Can you work these out from the model? Positions are in its coordinate system, mm. A direction names the side the tool comes from. Give positions to 0.01 mm unless a question says otherwise; leave off trailing zeros. Order: outer loops, then holes, each group sorted by start corner. A loop starts at its lowest first (then second) coordinate and runs counter-clockwise, first axis right, second up. Notation, with made-up numbers: (63.5, 84.5) - (116.5, 84.5) arc R20 ccw to (116.5, 99.5) - close; hole circle Ø1 at (65, -10). An arc over 180 degrees is marked (long way). Answer as CSV lines item,"result".
```python
from build123d import *

# Parameters (mm, degrees)
F0_W         = 35
F0_H         = 5
F1_DEPTH     = 1
F2_DEPTH     = 1.2
F3_W         = 5
F3_H         = 85
F4_DEPTH     = 2
F5_T4_DEPTH  = 99.1421356237
F5_T9_DEPTH  = 99.1421356237
F5_T14_DEPTH = 99.1421356237
F5_T19_DEPTH = 99.1421356237
F5_T24_DEPTH = 99.1421356237
F5_T29_DEPTH = 99.1421356237
F5_T34_DEPTH = 99.1421356237
F5_T39_DEPTH = 99.1421356237
F6_R         = 5


# Not quite as in the source:
# - a fillet or chamfer that OpenCascade refuses, or shapes differently, is made with other operations: its cross-section is extruded or revolved along the edge and cut away or added


with BuildPart() as f1:
    # F0 (on Top) → F1 (new body)
    with BuildSketch(Plane.XY):
        Polygon((-19.95, -49.95), (19.95, -49.95), (19.95, 49.95), (17.5, 49.95), (17.5, 44.95), (-17.5, 44.95), (-17.5, 49.95), (-19.95, 49.95), align=None)
        with Locations((0, 47.45)):
            Rectangle(F0_W, F0_H)
    extrude(amount=F1_DEPTH)

    # F0 (on Top) → F2 (join)
    with BuildSketch(Plane.XY):
        with Locations((0, 52.45)):
            Rectangle(F0_W, F0_H)
        with Locations((0, 47.45)):
            Rectangle(F0_W, F0_H)
    extrude(amount=-F2_DEPTH)

    # F3 (on face) → F4 (join)
    with BuildSketch(Plane.XY):
        with Locations((-12.45, 2.55)):
            Rectangle(F3_W, F3_H)
        with Locations((12.45, 2.55)):
            Rectangle(F3_W, F3_H)
    extrude(amount=-F4_DEPTH)

    # F5: fillet of radius 3 on 4 edges, made by hand


with BuildPart() as f5_tool2:
    # F5_s3 → F5_t4 (new body)
    with BuildSketch(Plane.XZ.offset(-52.1210678119)):
        with BuildLine():
            ThreePointArc((-14.95, 0), (-13.8536236828, -1.4494897428), (-12.1215728753, -2))
            Line((-12.1215728753, -2), (-14.95, -2))
            Line((-14.95, -2), (-14.95, 0))
        make_face()
    extrude(amount=F5_T4_DEPTH)

    split(bisect_by=Plane.XY.offset(-1.2), keep=Keep.BOTTOM)


with BuildPart() as f1_1:
    add(f1.part)

    # F5_t1: cut F5_tool2
    add(f5_tool2.part, mode=Mode.SUBTRACT)


with BuildPart() as f5_tool7:
    # F5_s8 → F5_t9 (new body)
    with BuildSketch(Plane.XZ.offset(-52.1210678119)):
        with BuildLine():
            ThreePointArc((-14.95, 0), (-13.8536236828, -1.4494897428), (-12.1215728753, -2))
            Line((-12.1215728753, -2), (-14.95, -2))
            Line((-14.95, -2), (-14.95, 0))
        make_face()
    extrude(amount=F5_T9_DEPTH)

    split(bisect_by=Plane.XZ.offset(-44.95), keep=Keep.TOP)


with BuildPart() as f1_2:
    add(f1_1.part)

    # F5_t6: cut F5_tool7
    add(f5_tool7.part, mode=Mode.SUBTRACT)


with BuildPart() as f5_tool12:
    # F5_s13 → F5_t14 (new body)
    with BuildSketch(Plane.XZ.offset(47.0210678119)):
        with BuildLine():
            ThreePointArc((-9.95, 0), (-11.0463763172, -1.4494897428), (-12.7784271247, -2))
            Line((-12.7784271247, -2), (-9.95, -2))
            Line((-9.95, -2), (-9.95, 0))
        make_face()
    extrude(amount=-F5_T14_DEPTH)

    split(bisect_by=Plane.XZ.offset(-44.95), keep=Keep.TOP)


with BuildPart() as f1_3:
    add(f1_2.part)

    # F5_t11: cut F5_tool12
    add(f5_tool12.part, mode=Mode.SUBTRACT)


with BuildPart() as f5_tool17:
    # F5_s18 → F5_t19 (new body)
    with BuildSketch(Plane.XZ.offset(47.0210678119)):
        with BuildLine():
            ThreePointArc((-9.95, 0), (-11.0463763172, -1.4494897428), (-12.7784271247, -2))
            Line((-12.7784271247, -2), (-9.95, -2))
            Line((-9.95, -2), (-9.95, 0))
        make_face()
    extrude(amount=-F5_T19_DEPTH)

    split(bisect_by=Plane.XY.offset(-1.2), keep=Keep.BOTTOM)


with BuildPart() as f1_4:
    add(f1_3.part)

    # F5_t16: cut F5_tool17
    add(f5_tool17.part, mode=Mode.SUBTRACT)


with BuildPart() as f5_tool22:
    # F5_s23 → F5_t24 (new body)
    with BuildSketch(Plane.XZ.offset(47.0210678119)):
        with BuildLine():
            ThreePointArc((14.95, 0), (13.8536236828, -1.4494897428), (12.1215728753, -2))
            Line((12.1215728753, -2), (14.95, -2))
            Line((14.95, -2), (14.95, 0))
        make_face()
    extrude(amount=-F5_T24_DEPTH)

    split(bisect_by=Plane.XZ.offset(-44.95), keep=Keep.TOP)


with BuildPart() as f1_5:
    add(f1_4.part)

    # F5_t21: cut F5_tool22
    add(f5_tool22.part, mode=Mode.SUBTRACT)


with BuildPart() as f5_tool27:
    # F5_s28 → F5_t29 (new body)
    with BuildSketch(Plane.XZ.offset(47.0210678119)):
        with BuildLine():
            ThreePointArc((14.95, 0), (13.8536236828, -1.4494897428), (12.1215728753, -2))
            Line((12.1215728753, -2), (14.95, -2))
            Line((14.95, -2), (14.95, 0))
        make_face()
    extrude(amount=-F5_T29_DEPTH)

    split(bisect_by=Plane.XY.offset(-1.2), keep=Keep.BOTTOM)


with BuildPart() as f1_6:
    add(f1_5.part)

    # F5_t26: cut F5_tool27
    add(f5_tool27.part, mode=Mode.SUBTRACT)


with BuildPart() as f5_tool32:
    # F5_s33 → F5_t34 (new body)
    with BuildSketch(Plane.XZ.offset(-52.1210678119)):
        with BuildLine():
            ThreePointArc((9.95, 0), (11.0463763172, -1.4494897428), (12.7784271247, -2))
            Line((12.7784271247, -2), (9.95, -2))
            Line((9.95, -2), (9.95, 0))
        make_face()
    extrude(amount=F5_T34_DEPTH)

    split(bisect_by=Plane.XY.offset(-1.2), keep=Keep.BOTTOM)


with BuildPart() as f1_7:
    add(f1_6.part)

    # F5_t31: cut F5_tool32
    add(f5_tool32.part, mode=Mode.SUBTRACT)


with BuildPart() as f5_tool37:
    # F5_s38 → F5_t39 (new body)
    with BuildSketch(Plane.XZ.offset(-52.1210678119)):
        with BuildLine():
            ThreePointArc((9.95, 0), (11.0463763172, -1.4494897428), (12.7784271247, -2))
            Line((12.7784271247, -2), (9.95, -2))
            Line((9.95, -2), (9.95, 0))
        make_face()
    extrude(amount=F5_T39_DEPTH)

    split(bisect_by=Plane.XZ.offset(-44.95), keep=Keep.TOP)


with BuildPart() as f1_8:
    add(f1_7.part)

    # F5_t36: cut F5_tool37
    add(f5_tool37.part, mode=Mode.SUBTRACT)

    # F6
    f6_edges = [f1_8.edges().sort_by_distance(p)[0] for p in [
        (-17.5, 54.95, -0.6),
        (17.5, 54.95, -0.6),
    ]]
    fillet(f6_edges, radius=F6_R)


solid = f1_8.part
```
1) I need wall thicknesses on line 1 along Y through (x, z) = (-5, -0.6); line 2 along Z through (x, y) = (6, -42.5); line 3 along Z through (x, y) = (13, 48). Which ranges of each line are inside material? Lowest first, please. Write a range as [from, to].
Answer block:
line 1,"[44.95, 54.95]"
line 2,"[0, 1]"
line 3,"[-1.2, 1]"
2) I want a section at D-D on z = 0.55. Write out the boundary of the cut face in (x, y), plus the area to 3 significant figures.
Answer block:
outline,"(-19.95, -49.95) - (19.95, -49.95) - (19.95, 49.95) - (-19.95, 49.95) - close"
area,"3,990 mm2"
3) I want a section at C-C on x = -8. Write out the boundary of the cut face in (y, z).
Answer block:
outline,"(-49.95, 0) - (44.95, 0) - (44.95, -1.2) - (54.95, -1.2) - (54.95, 0) - (49.95, 0) - (49.95, 1) - (-49.95, 1) - close"
4) Which directions (+Z, -Z, +X, -X, +Y, -Y) give clear straight access to the entire face, cutting with the end or side of a thin tool? Please do faces 1 (the cylindrical face through (14, 1.95, -1.34)), 2 (the flat face through (0, 52, 0)), 3 (the flat face through (-12, -39.95, -1)).
Answer block:
face 1,"-Z, +X, -Y"
face 2,"+Z, +X, -X, +Y"
face 3,"-Z, +X, -X, -Y"
5) I want a section at A-A on y = 30.5. Write out the boundary of the cut face in (x, z), plus the area to 3 significant figures.
Answer block:
outline,"(-19.95, 0) - (-14.95, 0) arc R3 ccw to (-12.45, -1.98) arc R3 ccw to (-9.95, 0) - (9.95, 0) arc R3 ccw to (12.45, -1.98) arc R3 ccw to (14.95, 0) - (19.95, 0) - (19.95, 1) - (-19.95, 1) - close"
area,"53.8 mm2"
6) I'm going to push flat-ended pins straight in: P1, Ø0.9, axis at x = -12, z = -2, coming from the +Y side; P2, Ø1.3, axis at x = -1.5, z = -1, coming from the -Y side; P3, Ø1, axis at x = 13.5, z = -1, coming from the -Y side; P4, Ø1.1, axis at x = 6, z = 0.5, coming from the +Y side. Where does each tip first touch, or does it pass through?
Answer block:
P1,"y = 45.05"
P2,"y = 44.95"
P3,"y = -39.95"
P4,"y = 54.95"
7) I want a section at B-B on x = -16.5. Write out the boundary of the cut face in (y, z).
Answer block:
outline,"(-49.95, 0) - (44.95, 0) - (44.95, -1.2) - (52.95, -1.2) - (52.95, 0) - (49.95, 0) - (49.95, 1) - (-49.95, 1) - close"
